For this review, take the finished solid that the model builds, in its own axes (mm). A direction names the side the tool comes from. Give positions to 0.01 mm unless a question says otherwise; leave off trailing zeros. Loops run counter-clockwise (first coordinate to the right, second up) from the corner with the lowest first, then second, coordinate; pieces in that order, holes last. Notation, with made-up numbers: (36.5, -20) -> (59.5, -20) arc R4 ccw to (59.5, -14) -> close; hole circle Ø11 at (68, 31). An arc over 180 degrees is marked (long way). Answer as CSV lines item,"result". Start each with the question number.
Item 1: Add section C-C on y = -12.5. State the section outline as (x, z) points.
Item 2: Add section D-D on z = 1. State the section outline as (x, y) points.
Item 3: Add section B-B on y = -21. State the section outline as (x, z) points.
Item 4: Machinability: for faces 1 (the face through (0, -11.5, 5)), 2 (the face through (4.96, -5.67, 15.83)), 3 (the face through (-3.55, -21, -8)), 4 (the face through (-8.8, -4.9, -10.4)), which of the approach directions +Z, -Z, +X, -X, +Y, -Y give a long, thin tool a straight path to every point of the face, cutting with its end or side? Answer none if there is none.
Item 5: Add section A-A on z = -5.75. State the section outline as (x, y) points, plus the area to 3 significant figures.
Item 6: Clearance check with flat-ended pins moving along their axes: P1, Ø9.5, axis at y = -17.5, z = 7, coming from the -X side; P2, Ø1.6, axis at x = 7.5, z = 5.5, coming from the -Y side; P3, Ø1.5, axis at x = -3.5, y = -10.5, coming from the -Z side; P4, Ø3, axis at x = 0, z = -9.5, coming from the +Y side. State where each tip first meets the part, or that it passes through.
Item 7: For L1, parallel to X at y = -12.7, z = 5.75; L2, parallel to X at y = -9, z = 4.5; L3, parallel to Z at x = 0.25, y = -10.5, list the stretches that pass through material, from the lowest coordinate up. Write a range as from..to.
Item 8: The part is to be moulded in two halves that separate along Z. For faces 5 (the face through (6, -13, -8)), 6 (the face through (0, -31.5, 0)), 7 (the face through (4.37, -4.93, -15.01)), say which applies: +Z half, -Z half, draft (parallel to the pull), parting line (faces both ways), or undercut.
```python
from build123d import *

# Parameters (mm, degrees)
ESBO_O1_W                = 26.7
ESBO_O1_H                = 39.3
RESSALTO_EXTRUS_O1_DEPTH = 38.5
CORTE_EXTRUS_O1_DEPTH    = 10
ESBO_O4_W                = 26.7
ESBO_O4_H                = 39.3
CORTE_EXTRUS_O2_DEPTH    = 10
ESBO_O5_W                = 26.7
ESBO_O5_H                = 39.3
ESBO_O5_W_2              = 22.6
ESBO_O5_H_2              = 27
CORTE_EXTRUS_O4_DEPTH    = 27
ESBO_O6_R                = 2.5
CORTE_EXTRUS_O5_DEPTH    = 5
ESBO_O7_W                = 2.05
ESBO_O7_H                = 1
RESSALTO_EXTRUS_O2_DEPTH = 4
CUT_EXTRUDE1_DEPTH       = 10
CUT_EXTRUDE1_DEPTH_BACK  = 100
SKETCH2_W                = 27
SKETCH2_H                = 27
ESBO_O4_3_W              = 26.7
ESBO_O4_3_H              = 39.3
CUT_EXTRUDE3_DEPTH       = 100
BOSS_EXTRUDE1_DEPTH      = 20
SKETCH6_3_W              = 5.45
SKETCH6_3_H              = 16
SKETCH6_3_R              = 1
BOSS_EXTRUDE2_DEPTH      = 2.4


with BuildPart() as part:
    # Esbo_o1 → Ressalto-extrus_o1 (new body)
    with BuildSketch(Plane(origin=(0, 0, 0), x_dir=(1, 0, 0), z_dir=(0, 1, 0))):
        Rectangle(ESBO_O1_W, ESBO_O1_H)
    extrude(amount=-RESSALTO_EXTRUS_O1_DEPTH)

    # Esbo_o2 → Corte-extrus_o1 (cut)
    with BuildSketch(Plane(origin=(0, 0, 0), x_dir=(1, 0, 0), z_dir=(0, 1, 0))):
        with BuildLine():
            Line((1.016622231, -18.102941176), (7.638740771, -11.999086257))
            ThreePointArc((7.638740771, -11.999086257), (8.829503459, -10.32964035), (9.25, -8.322615669))
            Line((9.25, -8.322615669), (9.25, 8.322615669))
            ThreePointArc((9.25, 8.322615669), (8.829503459, 10.32964035), (7.638740771, 11.999086257))
            Line((7.638740771, 11.999086257), (1.016622231, 18.102941176))
            ThreePointArc((1.016622231, 18.102941176), (0, 18.5), (-1.016622231, 18.102941176))
            Line((-1.016622231, 18.102941176), (-7.638740771, 11.999086257))
            ThreePointArc((-7.638740771, 11.999086257), (-8.829503459, 10.32964035), (-9.25, 8.322615669))
            Line((-9.25, 8.322615669), (-9.25, -8.322615669))
            ThreePointArc((-9.25, -8.322615669), (-8.829503459, -10.32964035), (-7.638740771, -11.999086257))
            Line((-7.638740771, -11.999086257), (-1.016622231, -18.102941176))
            ThreePointArc((-1.016622231, -18.102941176), (0, -18.5), (1.016622231, -18.102941176))
        make_face()
    extrude(amount=-CORTE_EXTRUS_O1_DEPTH, mode=Mode.SUBTRACT)

    # Esbo_o4 → Corte-extrus_o2 (cut)
    with BuildSketch(Plane(origin=(0, 0, 0), x_dir=(1, 0, 0), z_dir=(0, 1, 0))):
        Rectangle(ESBO_O4_W, ESBO_O4_H)
        with BuildLine():
            ThreePointArc((-8.316488925, 12.734380374), (-9.74540415, 10.731045286), (-10.25, 8.322615669))
            Line((-10.25, 8.322615669), (-10.25, -8.322615669))
            ThreePointArc((-10.25, -8.322615669), (-9.74540415, -10.731045286), (-8.316488925, -12.734380374))
            Line((-8.316488925, -12.734380374), (-1.694370386, -18.838235294))
            ThreePointArc((-1.694370386, -18.838235294), (0, -19.5), (1.694370386, -18.838235294))
            Line((1.694370386, -18.838235294), (8.316488925, -12.734380374))
            ThreePointArc((8.316488925, -12.734380374), (9.74540415, -10.731045286), (10.25, -8.322615669))
            Line((10.25, -8.322615669), (10.25, 8.322615669))
            ThreePointArc((10.25, 8.322615669), (9.74540415, 10.731045286), (8.316488925, 12.734380374))
            Line((8.316488925, 12.734380374), (1.694370386, 18.838235294))
            ThreePointArc((1.694370386, 18.838235294), (0, 19.5), (-1.694370386, 18.838235294))
            Line((-1.694370386, 18.838235294), (-8.316488925, 12.734380374))
        make_face(mode=Mode.SUBTRACT)
    extrude(amount=-CORTE_EXTRUS_O2_DEPTH, mode=Mode.SUBTRACT)

    # Esbo_o5 → Corte-extrus_o4 (cut)
    with BuildSketch(Plane.XZ.offset(38.5)):
        Rectangle(ESBO_O5_W, ESBO_O5_H)
        Rectangle(ESBO_O5_W_2, ESBO_O5_H_2, mode=Mode.SUBTRACT)
    extrude(amount=-CORTE_EXTRUS_O4_DEPTH, mode=Mode.SUBTRACT)

    # Esbo_o6 → Corte-extrus_o5 (cut)
    with BuildSketch(Plane(origin=(0, -10, 0), x_dir=(1, 0, 0), z_dir=(0, 1, 0))):
        with Locations(Location((0, -9.5, 0), (0, 0, 270))):
            Circle(ESBO_O6_R)
        with Locations(Location((0, 9.5, 0), (0, 0, 270))):
            Circle(ESBO_O6_R)
        with Locations(Location((-3, 0, 0), (0, 0, 270))):
            Circle(ESBO_O6_R)
    extrude(amount=-CORTE_EXTRUS_O5_DEPTH, mode=Mode.SUBTRACT)

    # Esbo_o7 → Ressalto-extrus_o2 (add)
    with BuildSketch(Plane.XZ.offset(11.5)):
        with Locations((12.325, 13)):
            Rectangle(ESBO_O7_W, ESBO_O7_H)
        with Locations((-12.325, 13)):
            Rectangle(ESBO_O7_W, ESBO_O7_H)
        with Locations((-12.325, -13)):
            Rectangle(ESBO_O7_W, ESBO_O7_H)
        with Locations((12.325, -13)):
            Rectangle(ESBO_O7_W, ESBO_O7_H)
    extrude(amount=RESSALTO_EXTRUS_O2_DEPTH)

    # Sketch2 → Cut-Extrude1 (cut, two sides: drawn at the far end of the back side and taken through both)
    with BuildSketch(Plane(origin=(11.3, 0, 0), x_dir=(0, 0, -1), z_dir=(1, 0, 0)).offset(-CUT_EXTRUDE1_DEPTH_BACK)):
        with Locations((0, -25)):
            Rectangle(SKETCH2_W, SKETCH2_H)
    extrude(amount=CUT_EXTRUDE1_DEPTH + CUT_EXTRUDE1_DEPTH_BACK, mode=Mode.SUBTRACT)

    # Esbo_o4_3 → Cut-Extrude3 (cut)
    with BuildSketch(Plane(origin=(0, 0, 0), x_dir=(1, 0, 0), z_dir=(0, 1, 0))):
        Rectangle(ESBO_O4_3_W, ESBO_O4_3_H)
        with BuildLine():
            ThreePointArc((-8.316488925, 12.734380374), (-9.74540415, 10.731045286), (-10.25, 8.322615669))
            Line((-10.25, 8.322615669), (-10.25, -8.322615669))
            ThreePointArc((-10.25, -8.322615669), (-9.74540415, -10.731045286), (-8.316488925, -12.734380374))
            Line((-8.316488925, -12.734380374), (-1.694370386, -18.838235294))
            ThreePointArc((-1.694370386, -18.838235294), (0, -19.5), (1.694370386, -18.838235294))
            Line((1.694370386, -18.838235294), (8.316488925, -12.734380374))
            ThreePointArc((8.316488925, -12.734380374), (9.74540415, -10.731045286), (10.25, -8.322615669))
            Line((10.25, -8.322615669), (10.25, 8.322615669))
            ThreePointArc((10.25, 8.322615669), (9.74540415, 10.731045286), (8.316488925, 12.734380374))
            Line((8.316488925, 12.734380374), (1.694370386, 18.838235294))
            ThreePointArc((1.694370386, 18.838235294), (0, 19.5), (-1.694370386, 18.838235294))
            Line((-1.694370386, 18.838235294), (-8.316488925, 12.734380374))
        make_face(mode=Mode.SUBTRACT)
    extrude(amount=-CUT_EXTRUDE3_DEPTH, mode=Mode.SUBTRACT)

    # Sketch6 → Boss-Extrude1 (add)
    with BuildSketch(Plane.XZ.offset(11.5)):
        with BuildLine():
            Line((-3.55, 13.2), (-3.55, 2.43874968))
            ThreePointArc((-3.55, 2.43874968), (-1.4387505, 1.952562419), (-0.5, 0))
            ThreePointArc((-0.5, 0), (-1.4387505, -1.952562419), (-3.55, -2.43874968))
            Line((-3.55, -2.43874968), (-3.55, -13.2))
            Line((-3.55, -13.2), (3.55, -13.2))
            Line((3.55, -13.2), (3.55, -8))
            Line((3.55, -8), (3.55, 8))
            Line((3.55, 8), (3.55, 13.2))
            Line((3.55, 13.2), (-3.55, 13.2))
        make_face()
        with BuildLine():
            Line((2.75, -12.4), (-2.75, -12.4))
            Line((-2.75, -12.4), (-2.75, -3.290516677))
            ThreePointArc((-2.75, -3.290516677), (-0.720448476, -2.386135967), (0.275667871, -0.4))
            Line((0.275667871, -0.4), (2.75, -0.4))
            Line((2.75, -0.4), (2.75, -12.4))
        make_face(mode=Mode.SUBTRACT)
        with BuildLine():
            Line((2.75, 12.4), (2.75, 0.4))
            Line((2.75, 0.4), (0.275667871, 0.4))
            ThreePointArc((0.275667871, 0.4), (-0.720448476, 2.386135967), (-2.75, 3.290516677))
            Line((-2.75, 3.290516677), (-2.75, 12.4))
            Line((-2.75, 12.4), (2.75, 12.4))
        make_face(mode=Mode.SUBTRACT)
    extrude(amount=BOSS_EXTRUDE1_DEPTH)

    # Sketch6_3 → Boss-Extrude2 (add)
    with BuildSketch(Plane.XZ.offset(11.5)):
        with Locations((6.275, 0)):
            Rectangle(SKETCH6_3_W, SKETCH6_3_H)
        with Locations(Location((7, 5.75, 0), (0, 0, 270))):
            Circle(SKETCH6_3_R, mode=Mode.SUBTRACT)
        with Locations(Location((7, -5.75, 0), (0, 0, 270))):
            Circle(SKETCH6_3_R, mode=Mode.SUBTRACT)
    extrude(amount=BOSS_EXTRUDE2_DEPTH)


solid = part.part
```
Computed values:
1,outline,"(-3.55, -13.2) -> (3.55, -13.2) -> (3.55, -8) -> (9, -8) -> (9, 8) -> (3.55, 8) -> (3.55, 13.2) -> (-3.55, 13.2) -> (-3.55, 2.44) arc R2.5 cw (long way) to (-3.55, -2.44) -> close; hole (-2.75, -12.4) -> (2.75, -12.4) -> (2.75, -0.4) -> (0.28, -0.4) arc R3.3 cw to (-2.75, -3.29) -> close; hole (-2.75, 3.29) arc R3.3 cw to (0.28, 0.4) -> (2.75, 0.4) -> (2.75, 12.4) -> (-2.75, 12.4) -> close; hole circle Ø2 at (7, -5.75); hole circle Ø2 at (7, 5.75)"
2,outline,"(-10.25, -11.5) -> (-5.29, -11.5) -> (-5.29, -10) -> (-9.25, -10) -> (-9.25, 0) -> (-10.25, 0) -> close; (-0.71, -31.5) -> (0.14, -31.5) -> (0.14, -11.5) -> (2.75, -11.5) -> (2.75, -31.5) -> (3.55, -31.5) -> (3.55, -13.9) -> (9, -13.9) -> (9, -11.5) -> (10.25, -11.5) -> (10.25, 0) -> (9.25, 0) -> (9.25, -10) -> (-0.71, -10) -> close"
3,outline,"(-3.55, -13.2) -> (3.55, -13.2) -> (3.55, 13.2) -> (-3.55, 13.2) -> (-3.55, 2.44) arc R2.5 cw (long way) to (-3.55, -2.44) -> close; hole (-2.75, -12.4) -> (2.75, -12.4) -> (2.75, -0.4) -> (0.28, -0.4) arc R3.3 cw to (-2.75, -3.29) -> close; hole (-2.75, 3.29) arc R3.3 cw to (0.28, 0.4) -> (2.75, 0.4) -> (2.75, 12.4) -> (-2.75, 12.4) -> close"
4,face 1,"-Y"
4,face 2,"+Z, +X, +Y, -Y"
4,face 3,"+Z, -Z, -X, -Y"
4,face 4,"+Y"
5,outline,"(-10.25, -11.5) -> (-3.55, -11.5) -> (-3.55, -31.5) -> (-2.75, -31.5) -> (-2.75, -11.5) -> (2.75, -11.5) -> (2.75, -31.5) -> (3.55, -31.5) -> (3.55, -13.9) -> (6, -13.9) -> (6, -11.5) -> (8, -11.5) -> (8, -13.9) -> (9, -13.9) -> (9, -11.5) -> (10.25, -11.5) -> (10.25, 0) -> (9.25, 0) -> (9.25, -10) -> (-9.25, -10) -> (-9.25, 0) -> (-10.25, 0) -> close"
5,area,"91.0 mm²"
6,P1,"x = -3.55"
6,P2,"y = -13.9"
6,P3,"z = -17.87"
6,P4,"through"
7,L1,"-3.55..-2.75, 2.75..6, 8..9"
7,L2,"-10.25..-9.25, 9.25..10.25"
7,L3,"-19.49..-11.99, -7.01..7.01, 11.99..19.49"
8,face 5,"-Z half"
8,face 6,"draft"
8,face 7,"undercut"
